from build123d import *

# Parameters (mm, degrees)
SKETCH1_W           = 34.5
SKETCH1_H           = 20
BOSS_EXTRUDE1_DEPTH = 2
SKETCH2_W           = 31.5
SKETCH2_H           = 5
BOSS_EXTRUDE2_DEPTH = 2
SKETCH3_W           = 3
SKETCH3_H           = 3
CUT_EXTRUDE1_DEPTH  = 10
FILLET1_R           = 2
CUT_EXTRUDE2_DEPTH  = 2


with BuildPart() as part:
    # Sketch1 → Boss-Extrude1 (new body)
    with BuildSketch(Plane.XY):
        Rectangle(SKETCH1_W, SKETCH1_H)
    extrude(amount=BOSS_EXTRUDE1_DEPTH)

    # Sketch2 → Boss-Extrude2 (add)
    with BuildSketch(Plane.XY.offset(2)):
        with Locations((0, 6)):
            Rectangle(SKETCH2_W, SKETCH2_H)
        with Locations((0, -6)):
            Rectangle(SKETCH2_W, SKETCH2_H)
    extrude(amount=BOSS_EXTRUDE2_DEPTH)

    # Sketch3 → Cut-Extrude1 (cut)
    with BuildSketch(Plane(origin=(0, 0, 0), x_dir=(-1, 0, 0), z_dir=(0, 0, -1))):
        with Locations((-4.25, -7)):
            Rectangle(SKETCH3_W, SKETCH3_H)
    extrude(amount=-CUT_EXTRUDE1_DEPTH, mode=Mode.SUBTRACT)

    # Fillet1
    # the kernel refuses this fillet: 2 mm, written as the material it takes off along each edge
    with BuildSketch(Plane(origin=(22.25, -10, 0), x_dir=(0, 1, 0), z_dir=(-1, 0, 0))) as fillet1_piece_1:
        with BuildLine():
            CenterArc((FILLET1_R, -FILLET1_R), FILLET1_R, 90, 90)
            Line((0, -FILLET1_R), (0, 0))
            Line((0, 0), (FILLET1_R, 0))
        make_face()
    extrude(amount=44.5, mode=Mode.SUBTRACT)
    with BuildSketch(Plane(origin=(-22.25, 10, 0), x_dir=(0, 0, 1), z_dir=(1, 0, 0))) as fillet1_piece_2:
        with BuildLine():
            CenterArc((FILLET1_R, FILLET1_R), FILLET1_R, 180, 90)
            Line((0, FILLET1_R), (0, 0))
            Line((0, 0), (FILLET1_R, 0))
        make_face()
    extrude(amount=44.5, mode=Mode.SUBTRACT)

    # Sketch4 → Cut-Extrude2 (cut)
    with BuildSketch(Plane.XY.offset(4)):
        Polygon((15.75, -8.5), (5.75, -8.5), (5.75, -5.5), (-12.75, -5.5), (-12.75, -3.5), (5.75, -3.5), (15.75, -3.5), align=None)
    extrude(amount=-CUT_EXTRUDE2_DEPTH, mode=Mode.SUBTRACT)


solid = part.part
Design review of the part built by this model. Coordinates are the model's own, in mm. A direction names the side the tool comes from. Round coordinates to 2 decimals unless told otherwise and drop trailing zeros. Write each loop counter-clockwise with the first axis right and the second up, starting at its lowest first coordinate (ties: lowest second). Pieces come first, ordered by that corner, then holes. Notation, with made-up numbers: (-36, -9.5) -> (8, -9.5) arc R22 cw to (8, 29.5) -> close; hole circle Ø11 at (-26.75, 20.25). An arc over 180 degrees is marked (long way). One line per item, written item: value. Start each with the question number.
Q1. Add section C-C (y = 6.5). Give the boundary of the cut face in (x, z), then the cut area to 3 significant figures.
Q2. Add section B-B (y = -6.75). Give the boundary of the cut face in (x, z).
Q3. The part is to be moulded in two halves that separate along Y. For faces 1 (the face through (0, 8.5, 3)), 2 (the face through (2.75, -7, 2)), 3 (the face through (17.25, 0, 1)), say which applies: pulls with the +Y half, pulls with the -Y half, needs draft (parallel to the pull), parting line crosses it, or undercut.
Q4. To check wall thickness, follow probe 1 along Y at (x, z) = (-3.5, 3.75); probe 2 along Z at (x, y) = (13.5, -2); probe 3 along Y at (x, z) = (13, 3.6). State the ranges of each line that lie inside material, in increasing order.
Q5. Tool access review of faces 4 (the face through (-5, -5.5, 3)), 5 (the face through (-15.75, 6, 3)), 6 (the face through (4, -5.5, 1)), 7 (the face through (0, 3.5, 3)): name each direction out of +Z, -Z, +X, -X, +Y, -Y from which nothing blocks a thin tool from reaching the whole face with its end or side.
Q6. Insertion check: P1, Ø0.6, axis at x = -5.5, z = 2.5, coming from the -Y side; P2, Ø0.6, axis at y = 6.5, z = 3.5, coming from the -X side; P3, Ø1, axis at y = -4.5, z = 3, coming from the +X side. Each pin has a flat end and moves straight along its axis. Give the tip position at first contact, or say it passes through.
Q7. Add section A-A (z = 3.55). Give the boundary of the cut face in (x, y), then the cut area to 3 significant figures.
Q8. Add section D-D (x = -7). Give the boundary of the cut face in (y, z), then the cut area to 3 significant figures.
Response:
1. outline: (-17.25, 0) -> (17.25, 0) -> (17.25, 2) -> (15.75, 2) -> (15.75, 4) -> (-15.75, 4) -> (-15.75, 2) -> (-17.25, 2) -> close
1. area: 132 mm^2
2. outline: (-17.25, 0) -> (2.75, 0) -> (2.75, 4) -> (-15.75, 4) -> (-15.75, 2) -> (-17.25, 2) -> close; (5.75, 0) -> (17.25, 0) -> (17.25, 2) -> (5.75, 2) -> close
3. face 1: pulls with the +Y half
3. face 2: undercut
3. face 3: needs draft
4. probe 1: y = -8.5 to -5.5, 3.5 to 8.5
4. probe 2: z = 0 to 2
4. probe 3: y = 3.5 to 8.5
5. face 4: +Z, +X
5. face 5: +Z, -X, +Y, -Y
5. face 6: +Z, -Z
5. face 7: +Z, +X, -X
6. P1: stops at y = -8.5
6. P2: stops at x = -15.75
6. P3: stops at x = -12.75
7. outline: (-15.75, -8.5) -> (2.75, -8.5) -> (2.75, -5.5) -> (-12.75, -5.5) -> (-12.75, -3.5) -> (-15.75, -3.5) -> close; (-15.75, 3.5) -> (15.75, 3.5) -> (15.75, 8.5) -> (-15.75, 8.5) -> close
7. area: 219 mm^2
8. outline: (-10, 2) arc R2 ccw to (-8, 0) -> (8, 0) arc R2 ccw to (10, 2) -> (8.5, 2) -> (8.5, 4) -> (3.5, 4) -> (3.5, 2) -> (-5.5, 2) -> (-5.5, 4) -> (-8.5, 4) -> (-8.5, 2) -> close
8. area: 54.3 mm^2
